```python
from build123d import *

# Parameters (mm, degrees)
PAD_DEPTH     = 18
SKETCH001_R   = 7.5
SKETCH001_R_2 = 4
PAD001_DEPTH  = 15


with BuildPart() as part:
    # Sketch → Pad (new body)
    with BuildSketch(Plane(origin=(0, 0, 0), x_dir=(0.939693, -0.34202, 0), z_dir=(0, 0, 1))):
        Polygon((-5.25, 20), (-5.25, 0), (5.25, 0), (5.25, 20), (3.25, 20), (3.25, 2), (-3.25, 2), (-3.25, 20), align=None)
    extrude(amount=PAD_DEPTH)

    # Sketch001 → Pad001 (join)
    with BuildSketch(Plane.YZ):
        Polygon((12.727922, 18), (5.272078, 18), (0, 12.727922), (0, 5.272078), (5.272078, 0), (12.727922, 0), (18, 5.272078), (18, 12.727922), align=None)
        with Locations((9, 9)):
            Circle(SKETCH001_R, mode=Mode.SUBTRACT)
        with Locations((9, 9)):
            Circle(SKETCH001_R_2)
    extrude(amount=-PAD001_DEPTH)


solid = part.part
```
Geometry: final body of the model. Coordinates: model frame, mm. A direction names the side the tool comes from. Round coordinates to 2 decimals unless told otherwise and drop trailing zeros. Loops run counter-clockwise (first coordinate to the right, second up) from the corner with the lowest first, then second, coordinate; pieces in that order, holes last. Notation, with made-up numbers: (85.25, 27) -> (95.25, 27) arc R24 ccw to (95.25, 66) -> close; hole circle Ø3 at (29, 53.25). An arc over 180 degrees is marked (long way). Use one line per item in the form item = value. Start each with the question number.
1) Section D-D on y = 4. Output: boundary loops of the cut face in (x, z), then the cut area to 3 significant figures.
2) Section B-B on z = 9. Output: boundary loops of the cut face in (x, y).
3) Line query: L1, parallel to Z at x = -5.5, y = 9; L2, parallel to X at y = 16, z = 5.75. Output: solid intervals per line, ascending.
4) Access query for faces 1 (the cylindrical face through (-7.829, 12.815, 10.201)), 2 (the flat face through (-0.91, 3.72, 16.45)), 3 (the flat face through (0, 5.5, 1.9)), 4 (the flat face through (-7.4, 15.4, 15.33)). Directions: +Z, -Z, +X, -X, +Y, -Y. A direction counts if a zero-diameter tool reaches every point of the face in a straight line with its end or side. Return the directions, or none.
5) Section A-A on x = -6.75. Output: boundary loops of the cut face in (y, z), then the cut area to 3 significant figures.
6) First-contact query: P1, Ø5, axis at y = 7.5, z = 9.5, coming from the +X side; P2, Ø1, axis at y = 7, z = 13.5, coming from the -X side; P3, Ø2, axis at y = 7, z = 4.5, coming from the +X side. Flat tips, straight axial feed; report the tip coordinate or a pass-through.
7) Section C-C on y = 9. Output: boundary loops of the cut face in (x, z).
8) Draft query along X for faces 5 (the flat face through (10.847, 17.335, 8.874)), 6 (the flat face through (-7, 0, 9)), 7 (the flat face through (-2.145, 3.609, 17.35)). Return one class per face: released by +X, released by -X, zero draft, split by the parting line, or undercut.
Response:
q1.outline = (-15, 1.27) -> (-4.13, 1.27) -> (-4.13, 0) -> (-2, 0) -> (-2, 1.27) -> (0, 1.27) -> (0, 3.41) -> (-2, 3.41) -> (-2, 14.59) -> (0, 14.59) -> (0, 16.73) -> (-2, 16.73) -> (-2, 18) -> (-4.13, 18) -> (-4.13, 16.73) -> (-15, 16.73) -> (-15, 14.59) -> (-4.13, 14.59) -> (-4.13, 3.41) -> (-15, 3.41) -> close; (4.91, 0) -> (7.04, 0) -> (7.04, 18) -> (4.91, 18) -> close
q1.area = 132 mm^2
q2.outline = (-15, 0) -> (0, 0) -> (4.93, -1.8) -> (11.77, 17) -> (9.89, 17.68) -> (3.74, 0.77) -> (-2.37, 2.99) -> (-1.64, 5) -> (0, 5) -> (0, 9.5) -> (3.79, 19.91) -> (1.91, 20.59) -> (-0.86, 13) -> (-15, 13) -> (-15, 5) -> (-3.77, 5) -> (-4.93, 1.8) -> (-4.12, 1.5) -> (-15, 1.5) -> close; (-15, 16.5) -> (0, 16.5) -> (0, 18) -> (-15, 18) -> close
q3.L1 = 0 to 1.5, 5 to 13, 16.5 to 18
q3.L2 = -15 to 0, 0.24 to 2.36, 9.28 to 11.41
q4.face_1 = -X
q4.face_2 = +Z
q4.face_3 = +Z, -Z
q4.face_4 = +Z, -X, +Y
q5.outline = (0, 5.27) -> (5.27, 0) -> (12.73, 0) -> (18, 5.27) -> (18, 12.73) -> (12.73, 18) -> (5.27, 18) -> (0, 12.73) -> close; circle Ø8 at (9, 9); hole circle Ø15 at (9, 9)
q5.area = 142 mm^2
q6.P1 = 9.23
q6.P2 = -3.22
q6.P3 = 8.5
q7.outline = (-15, 0) -> (0, 0) -> (0, 1.5) -> (-0.18, 1.5) -> (-0.18, 5) -> (0, 5) -> (0, 13) -> (-0.18, 13) -> (-0.18, 16.5) -> (0, 16.5) -> (0, 18) -> (-15, 18) -> (-15, 16.5) -> (-2.31, 16.5) -> (-2.31, 13) -> (-15, 13) -> (-15, 5) -> (-2.31, 5) -> (-2.31, 1.5) -> (-15, 1.5) -> close; (6.73, 0) -> (8.86, 0) -> (8.86, 18) -> (6.73, 18) -> close
q8.face_5 = released by +X
q8.face_6 = zero draft
q8.face_7 = undercut
